Could you check a few things on this drawing? It's one solid part, dimensions in mm from its lowest x, y, z. Give positions to 0.01 mm unless a question says otherwise; leave off trailing zeros. Write each loop counter-clockwise with the first axis right and the second up, starting at its lowest first coordinate (ties: lowest second). Pieces come first, ordered by that corner, then holes. Notation, with made-up numbers: (-4.5, 46) -> (41.5, 46) arc R6 ccw to (41.5, 50) -> close; hole circle Ø2 at (19, 7). An arc over 180 degrees is marked (long way). Answer as CSV lines item,"result". Start each with the question number.
1. If we section it at A-A on z = 3.75: Write out the boundary of the cut face in (x, y), plus the area to 3 significant figures.
2. I'm going to push a flat-ended pin straight in: P1, Ø4, axis at y = 4.5, z = 2, coming from the -X side. Where does the tip first touch, or does it pass through?
3. If we section it at B-B on y = 1: Write out the boundary of the cut face in (x, z).
4. I need wall thicknesses on line 1 (X direction, y = 2, z = 4); line 2 (X direction, y = 3.75, z = 5.25). Which ranges of each line are inside material? Lowest first, please. Write a range as [from, to].
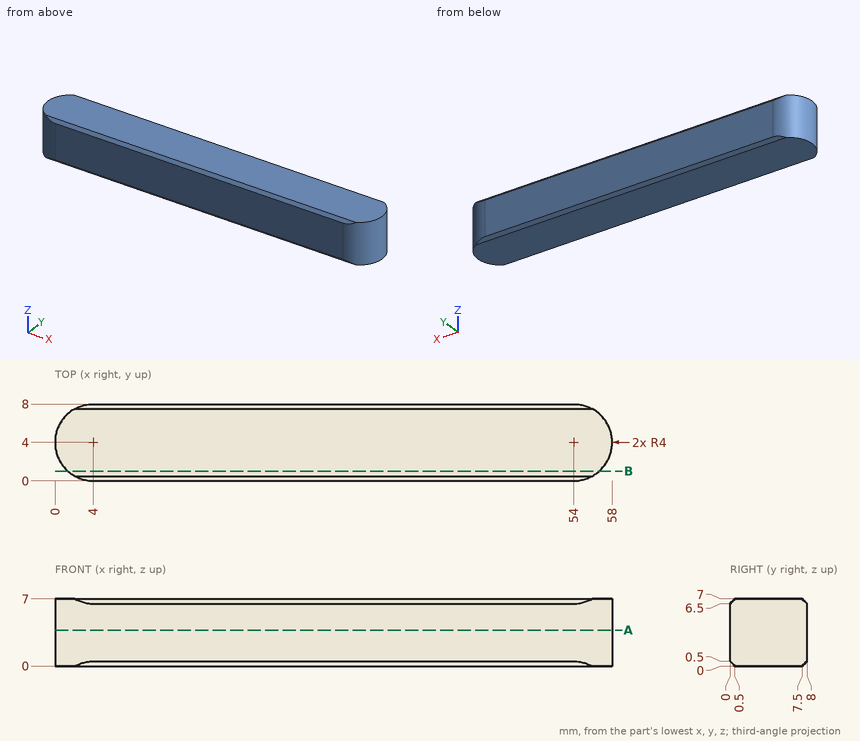
Computed values:
1,outline,"(4, 0) -> (54, 0) arc R4 ccw to (54, 8) -> (4, 8) arc R4 ccw to start"
1,area,"450 mm2"
2,P1,"stops at x = 0"
3,outline,"(1.35, 0) -> (56.65, 0) -> (56.65, 7) -> (1.35, 7) -> close"
4,line 1,"x = [0.54, 57.46]"
4,line 2,"x = [0.01, 57.99]"
